```python
from build123d import *

# Parameters (mm, degrees)
F0_W     = 76.2
F0_H     = 76.2
F1_DEPTH = 38.1
F2_DEPTH = 38.1
F3_T     = -7.62
F4_SIZE  = 5.08
F5_SIZE  = 5.08


with BuildPart() as f1:
    # F0 (on Front) → F1 (new body)
    with BuildSketch(Plane.XZ):
        Rectangle(F0_W, F0_H)
    extrude(amount=F1_DEPTH)

    # F2 (add): a face of the model
    f2_faces = [f1.faces().sort_by_distance(p)[0] for p in [
        (0, 0, 0),
    ]]
    extrude(f2_faces, amount=F2_DEPTH)

    # F3
    f3_openings = [f1.faces().sort_by_distance(p)[0] for p in [
        (0, 0, 38.1),
    ]]
    offset(amount=F3_T, openings=f3_openings)

    # F4
    f4_edges = [f1.edges().sort_by_distance(p)[0] for p in [
        (-30.48, 0, 38.1),
        (0, -30.48, 38.1),
        (0, 30.48, 38.1),
        (30.48, 0, 38.1),
    ]]
    chamfer(f4_edges, length=F4_SIZE)

    # F5
    f5_edges = [f1.edges().sort_by_distance(p)[0] for p in [
        (0, 30.48, -30.48),
        (-30.48, 0, -30.48),
        (30.48, 0, -30.48),
        (0, -30.48, -30.48),
    ]]
    chamfer(f5_edges, length=F5_SIZE)


solid = f1.part
```
Read the model definition and answer for the solid it produces. Units are mm, in the model's axes. A direction names the side the tool comes from. Give positions to 0.01 mm unless a question says otherwise; leave off trailing zeros. Order: outer loops, then holes, each group sorted by start corner. A loop starts at its lowest first (then second) coordinate and runs counter-clockwise, first axis right, second up. Notation, with made-up numbers: (70.5, 68) -> (100.5, 68) arc R28 cw to (100.5, 107) -> close; hole circle Ø2 at (56.25, 27.5). An arc over 180 degrees is marked (long way). One line per item, written item: value. Start each with the question number.
(1) The part is cut by section D-D (y = -32.5). Determine the outline of the cut face in (x, z), and give its area (3 significant figures).
(2) For a pull along X with two mould halves and no side action, classify faces 3 (the flat face through (-3, 37, 38.1)), 4 (the flat face through (-0.43, 27.9, -27.98)), 5 (the flat face through (-27.9, -0.43, -27.98)), 6 (the flat face through (-38.1, -1, -1)) as released by +X, released by -X, zero draft, split by the parting line, or undercut.
(3) The part is cut by section C-C (x = -5.5). Determine the outline of the cut face in (y, z).
(4) Straight lines are drawn through the part: L1, parallel to X at y = -28, z = -25; L2, parallel to X at y = -29, z = 33.5. For each, find the intervals that lie inside material, in ascending order.
(5) The part is cut by section B-B (z = 14). Determine the outline of the cut face in (x, y).
(6) A tool of negligible diameter and unlimited length cuts with its end or side. For faces 1 (the flat face through (38.1, -1, -1)), 2 (the flat face through (-0.5, 32.98, 35.52)), from which of +Z, -Z, +X, -X, +Y, -Y can it reach the whole face along a straight path? Write none if from no direction.
(7) The part is cut by section A-A (y = 33.5). Determine the outline of the cut face in (x, z).
Taken from the geometry:
1. outline: (-38.1, -38.1) -> (38.1, -38.1) -> (38.1, 38.1) -> (35.56, 38.1) -> (32.5, 35.04) -> (-32.5, 35.04) -> (-35.56, 38.1) -> (-38.1, 38.1) -> close
1. area: 5,600 mm^2
2. face 3: zero draft
2. face 4: undercut
2. face 5: undercut
2. face 6: released by -X
3. outline: (-38.1, -38.1) -> (38.1, -38.1) -> (38.1, 38.1) -> (35.56, 38.1) -> (30.48, 33.02) -> (30.48, -25.4) -> (25.4, -30.48) -> (-25.4, -30.48) -> (-30.48, -25.4) -> (-30.48, 33.02) -> (-35.56, 38.1) -> (-38.1, 38.1) -> close
4. L1: -38.1 to -30.48, 30.48 to 38.1
4. L2: -38.1 to -30.96, 30.96 to 38.1
5. outline: (-38.1, -38.1) -> (38.1, -38.1) -> (38.1, 38.1) -> (-38.1, 38.1) -> close; hole (-30.48, -30.48) -> (30.48, -30.48) -> (30.48, 30.48) -> (-30.48, 30.48) -> close
6. face 1: +Z, -Z, +X, +Y, -Y
6. face 2: +Z
7. outline: (-38.1, -38.1) -> (38.1, -38.1) -> (38.1, 38.1) -> (35.56, 38.1) -> (33.5, 36.04) -> (-33.5, 36.04) -> (-35.56, 38.1) -> (-38.1, 38.1) -> close
